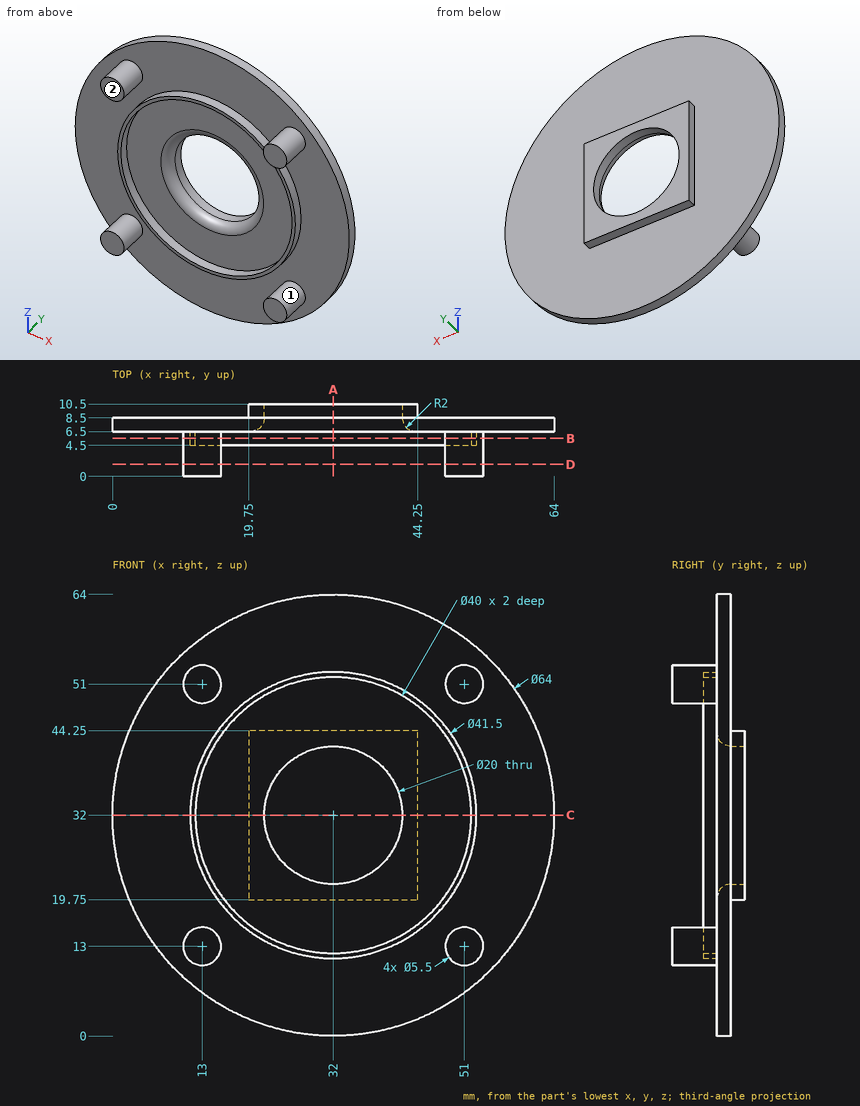
Drawing for the job (mm, zero at the part's lowest x, y, z). A direction names the side the tool comes from. Give positions to 0.01 mm unless a question says otherwise; leave off trailing zeros. Order: outer loops, then holes, each group sorted by start corner. A loop starts at its lowest first (then second) coordinate and runs counter-clockwise, first axis right, second up. Notation, with made-up numbers: M 14,-22 L 65,-22 A35 ccw 65,11 Z; hole C 8,16 d2. An arc over 180 degrees is marked long. Use a Markdown table: item, result. Add a question column.
(1) Probe line 1 along X through (y, z) = (9.7, 32); line 2 along Y through (x, z) = (53, 34). List the from-to ranges inside material, lowest first. Write a range as [from, to].
(2) Saw through at A-A, the plane x = 32. Give the cut face in (y, z), and give its area (3 significant figures).
(3) Drop flat-ended pins along their axis: P1, Ø2, axis at x = 27.5, y = 4.5, coming from the -Z side; P2, Ø2, axis at x = 29.5, y = 5, coming from the +Z side; P3, Ø5, axis at x = 46.5, y = 3, coming from the +Z side; P4, Ø24, axis at x = 32, z = 32, coming from the +Y side. Give the stop position or say it passes through.
(4) Saw through at D-D, the plane y = 1.75. Give the cut face in (x, z), and give its area (3 significant figures).
(5) Saw through at C-C, the plane z = 32. Give the cut face in (x, y), and give its area (3 significant figures).
(6) Saw through at B-B, the plane y = 5.5. Give the cut face in (x, z), and give its area (3 significant figures).
(7) 3-axis set-ups, long thin cutter, end or side, ignore diameter. For the marked faces 1 and 2: which of +Z, -Z, +X, -X, +Y, -Y reach the whole face in a straight line?
Answer key:
| question | item | result |
|---|---|---|
| 1 | line 1 | [19.75, 22], [42, 44.25] |
| 1 | line 2 | [6.5, 8.5] |
| 2 | outline | M 4.5,11.25 L 6.5,11.25 L 6.5,0 L 8.5,0 L 8.5,19.75 L 10.5,19.75 L 10.5,22 L 8.5,22 A2 ccw 6.5,20 L 6.5,12 L 4.5,12 Z; M 4.5,52 L 6.5,52 L 6.5,44 A2 ccw 8.5,42 L 10.5,42 L 10.5,44.25 L 8.5,44.25 L 8.5,64 L 6.5,64 L 6.5,52.75 L 4.5,52.75 Z |
| 2 | area | 98.3 mm^2 |
| 3 | P1 | z = 11.55 |
| 3 | P2 | z = 52.7 |
| 3 | P3 | z = 52.89 |
| 3 | P4 | y = 10.5 |
| 4 | outline | C 13,13 d5.5; C 13,51 d5.5; C 51,13 d5.5; C 51,51 d5.5 |
| 4 | area | 95.0 mm^2 |
| 5 | outline | M 0,6.5 L 11.25,6.5 L 11.25,4.5 L 12,4.5 L 12,6.5 L 20,6.5 A2 ccw 22,8.5 L 22,10.5 L 19.75,10.5 L 19.75,8.5 L 0,8.5 Z; M 42,8.5 A2 ccw 44,6.5 L 52,6.5 L 52,4.5 L 52.75,4.5 L 52.75,6.5 L 64,6.5 L 64,8.5 L 44.25,8.5 L 44.25,10.5 L 42,10.5 Z |
| 5 | area | 98.3 mm^2 |
| 6 | outline | C 13,13 d5.5; C 13,51 d5.5; C 32,32 d41.5; C 51,13 d5.5; C 51,51 d5.5; hole C 32,32 d40 |
| 6 | area | 191 mm^2 |
| 7 | face 1 | -Y |
| 7 | face 2 | +Z, -Z, +X, -X, -Y |
